from build123d import *


with BuildPart() as part:
    # Sketch1 → Revolve1 (revolve)
    with BuildSketch(Plane.XY):
        Polygon((6.35, -2.195764302), (63.5, -2.195764302), (90.440768363, 24.745004061), (90.440768363, 39.985004061), (80.280768363, 39.985004061), (80.280768363, 45.065004061), (90.440768363, 45.065004061), (90.440768363, 50.145004061), (80.280768363, 50.145004061), (80.280768363, 55.225004061), (90.440768363, 55.225004061), (90.440768363, 159.365004061), (63.5, 186.305772424), (12.7, 186.305772424), (12.7, 237.105772424), (0, 237.105772424), (0, 0), (0, -25.4650148), (6.35, -25.4650148), align=None)
        Polygon((22.967294816, 176.145772424), (62.500768363, 176.145772424), (80.280768363, 158.365772424), (80.280768363, 140.585772424), (12.807294816, 140.585772424), (12.807294816, 165.985772424), (22.967294816, 165.985772424), align=None, mode=Mode.SUBTRACT)
    revolve(axis=Axis((0, 237.105772424, 0), (0, 1, 0)))


solid = part.part
The model under review builds one solid part; all positions refer to its coordinate system, in mm. A direction names the side the tool comes from. Round coordinates to 2 decimals unless told otherwise and drop trailing zeros. Loops run counter-clockwise (first coordinate to the right, second up) from the corner with the lowest first, then second, coordinate; pieces in that order, holes last. Notation, with made-up numbers: (-9, 14) - (-4, 14) arc R21 ccw to (-4, 47) - close; hole circle Ø6 at (82, 65.25). An arc over 180 degrees is marked (long way). Use CSV: the item, a comma, the result in double quotes.
(1) The part is to be moulded in two halves that separate along X. For faces 1 (the flat face through (1, 176.146, 27)), 2 (the cylindrical face through (-11.77, 47.64, -89.67)), 3 (the flat face through (-34, 39.985, 73)), say which applies: pulls with the +X half, pulls with the -X half, needs draft (parallel to the pull), parting line crosses it, or undercut.
Working result:
face 1,"undercut"
face 2,"parting line crosses it"
face 3,"needs draft"
(2) Clearance check with flat-ended pins moving along their axes: P1, Ø1.5, axis at x = 12, z = -55.5, coming from the +Y side; P2, Ø1.5, axis at y = 121, z = 44, coming from the -X side; P3, Ø1.5, axis at x = 55.5, y = 167, coming from the -Z side; P4, Ø1, axis at y = 186, z = -65, coming from the -X side. State where each tip first meets the part, or that it passes through.
Working result:
P1,"stops at y = 186.31"
P2,"stops at x = -79.43"
P3,"stops at z = -62.66"
P4,"passes through"
(3) Take a section at D-D, the plane y = 130. Give the boundary of the cut face in (x, z), plus the area to 3 significant figures.
Working result:
outline,"circle Ø180.88 at (0, 0)"
area,"25,700 mm^2"
(4) Take a section at A-A, the plane x = 0. State how many separate pieces and enclosed holes the cut face has, plus the area to 3 significant figures.
Working result:
separate pieces,"1"
enclosed holes,"2"
area,"29,700 mm^2"
(5) Take a section at C-C, the plane y = 202.5. Give the boundary of the cut face in (x, z), plus the area to 3 significant figures.
Working result:
outline,"circle Ø25.4 at (0, 0)"
area,"507 mm^2"
(6) For line 1 (Z direction, x = 0, y = 145.5); line 2 (Y direction, x = -3.5, z = 60), list the stretches that pass through material, from the lowest coordinate up.
Working result:
line 1,"z = -90.44 to -80.28, -12.81 to 12.81, 80.28 to 90.44"
line 2,"y = -2.2 to 140.59, 176.15 to 186.31"
(7) Machinability: for faces 4 (the cylindrical face through (-2.75, 212.06, 12.4)), 5 (the conical face through (-14.131, -0.51, 63.635)), 6 (the flat face through (34, 55.225, 73)), which of the approach directions +Z, -Z, +X, -X, +Y, -Y give a long, thin tool a straight path to every point of the face, cutting with its end or side? Answer none if there is none.
Working result:
face 4,"+Y"
face 5,"-Y"
face 6,"none"
